For this review, take the finished solid that the model builds, in its own axes (mm). Round coordinates to 2 decimals unless told otherwise and drop trailing zeros. Order: outer loops, then holes, each group sorted by start corner. A loop starts at its lowest first (then second) coordinate and runs counter-clockwise, first axis right, second up. Notation, with made-up numbers: (9.25, 61.5) - (52.25, 61.5) arc R16 ccw to (52.25, 87.5) - close; hole circle Ø5 at (76, 6.25). An arc over 180 degrees is marked (long way). One line per item, written item: value.
```python
from build123d import *

# Parameters (mm, degrees)
F0_W     = 150
F0_H     = 150
F0_W_2   = 130
F0_H_2   = 130
F1_DEPTH = 4
F3_DEPTH = 4


with BuildPart() as f1:
    # F0 (on Top) → F1 (new body)
    with BuildSketch(Plane.XY):
        Rectangle(F0_W, F0_H)
        Rectangle(F0_W_2, F0_H_2, mode=Mode.SUBTRACT)
    extrude(amount=F1_DEPTH)

    # F2 (on Top) → F3 (join, through all)
    with BuildSketch(Plane.XY):
        Polygon((-35, 10), (-65, 10), (-65, 5), (-40, 5), (-40, -5), (-65, -5), (-65, -10), (-35, -10), align=None)
        Polygon((-5, 65), (-10, 65), (-10, 35), (10, 35), (10, 65), (5, 65), (5, 40), (-5, 40), align=None)
        Polygon((65, 5), (65, 10), (35, 10), (35, -10), (65, -10), (65, -5), (40, -5), (40, 5), align=None)
        Polygon((5, -65), (10, -65), (10, -35), (-10, -35), (-10, -65), (-5, -65), (-5, -40), (5, -40), align=None)
    extrude(amount=F3_DEPTH)


solid = f1.part
```
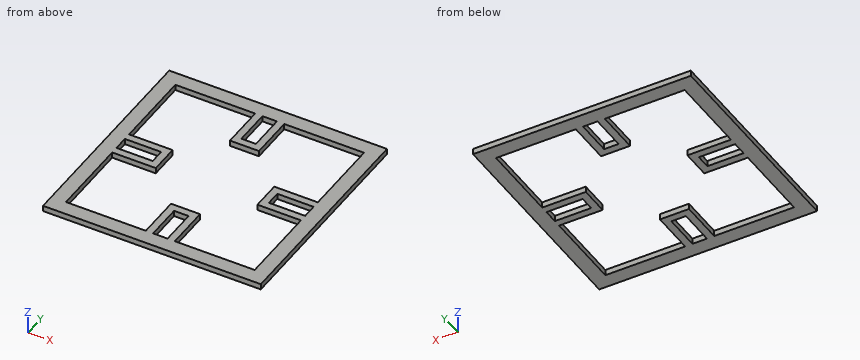
Item 1: Wall thickness on line 1 (Y direction, x = -50, z = 0.5); line 2 (X direction, y = -38, z = 0.3); line 3 (Y direction, x = 4, z = 0.85): over which ranges is each line inside the solid? List them lowest first.
Returned:
line 1: -75 to -65, -10 to -5, 5 to 10, 65 to 75
line 2: -75 to -65, -10 to 10, 65 to 75
line 3: -75 to -65, -40 to -35, 35 to 40, 65 to 75
Item 2: Take a section at A-A (y = 28). Write out the cut boundary in (x, z).
Returned:
outline: (-75, 0) - (-65, 0) - (-65, 4) - (-75, 4) - close; (65, 0) - (75, 0) - (75, 4) - (65, 4) - close
Item 3: Take a section at C-C (y = 55.5). Write out the cut boundary in (x, z), plus the area to 3 significant figures.
Returned:
outline: (-75, 0) - (-65, 0) - (-65, 4) - (-75, 4) - close; (-10, 0) - (-5, 0) - (-5, 4) - (-10, 4) - close; (5, 0) - (10, 0) - (10, 4) - (5, 4) - close; (65, 0) - (75, 0) - (75, 4) - (65, 4) - close
area: 120 mm^2
